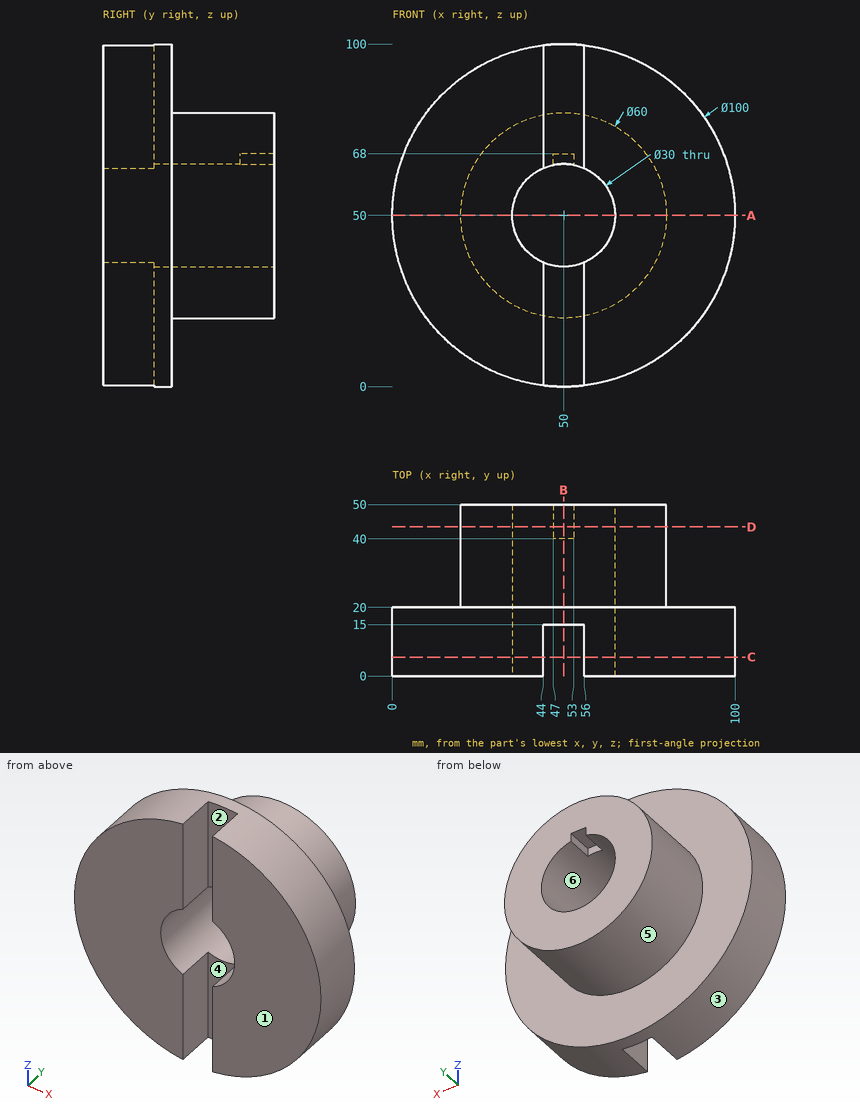
Input: dimensioned drawing with shaded views. Units: mm. Origin: part minimum x, y, z. A direction names the side the tool comes from. Coordinates: 2 decimals unless noted, no trailing zeros. Order: outer loops, then holes, each group sorted by start corner. A loop starts at its lowest first (then second) coordinate and runs counter-clockwise, first axis right, second up. Notation, with made-up numbers: (20.25, 61.25) - (76.25, 61.25) arc R9 cw to (76.25, 70.25) - close; hole circle Ø6 at (-17.75, -33). An arc over 180 degrees is marked (long way). Return JSON: item names as keys, results as strings. Group by question number.
1. Cut plane C-C (y = 5.5). Output: boundary loops of the cut face in (x, z).
2. Material intervals for line 1 along Z through (x, y) = (50, 21.5); line 2 along X through (y, z) = (9.5, 25); line 3 along Y through (x, z) = (50, 7), sorted ascending. Write a range as [from, to].
3. Cut plane A-A (z = 50). Output: boundary loops of the cut face in (x, y).
4. Cut plane D-D (y = 43.5). Output: boundary loops of the cut face in (x, z).
5. Set-up query: the marked faces 4, 5 and 6. Return all of +Z, -Z, +X, -X, +Y, -Y with unobstructed straight access to the full face (end or side cutting, diameter ignored); none if empty.
6. Pin query (flat end, axial travel): pin 1 (1 mm diameter, centred on y = 42.5, z = 66.5, fed in from -X); pin 2 (3 mm diameter, centred on y = 12.5, z = 83, fed in from -X); pin 3 (8 mm diameter, centred on x = 16.5, y = 8.5, fed in from +Z); pin 4 (3 mm diameter, centred on x = 62, z = 46, fed in from +Y). Return the tip coordinate at first contact, or that it passes through.
7. Cut plane B-B (x = 50). Output: boundary loops of the cut face in (y, z).
8. Pull-direction query (X, two-part tool) for the marked faces 1, 2 and 3; classes: pulls with the +X half, pulls with the -X half, needs draft (parallel to the pull), parting line crosses it, or undercut.
Resolved:
{
 "1": {"outline": "(44, 0.36) - (44, 36.25) arc R15 cw to (44, 63.75) - (44, 99.64) arc R50 ccw to start; (56, 0.36) arc R50 ccw to (56, 99.64) - (56, 63.75) arc R15 cw to (56, 36.25) - close"},
 "2": {"line 1": "z = [20, 35], [65, 80]", "line 2": "x = [6.7, 44], [56, 93.3]", "line 3": "y = [15, 20]"},
 "3": {"outline": "(0, 0) - (35, 0) - (35, 50) - (20, 50) - (20, 20) - (0, 20) - close; (65, 0) - (100, 0) - (100, 20) - (80, 20) - (80, 50) - (65, 50) - close"},
 "4": {"outline": "circle Ø60 at (50, 50); hole (47, 64.7) arc R15 ccw (long way) to (53, 64.7) - (53, 68) - (47, 68) - close"},
 "5": {"face 4": "+Z, -Z, -Y", "face 5": "+Y", "face 6": "+Y, -Y"},
 "6": {"pin 1": "stops at x = 24.62", "pin 2": "stops at x = 11.17", "pin 3": "stops at z = 90.37", "pin 4": "passes through"},
 "7": {"outline": "(15, 0) - (20, 0) - (20, 20) - (50, 20) - (50, 35) - (15, 35) - close; (15, 65) - (40, 65) - (40, 68) - (50, 68) - (50, 80) - (20, 80) - (20, 100) - (15, 100) - close"},
 "8": {"face 1": "needs draft", "face 2": "undercut", "face 3": "parting line crosses it"}
}
